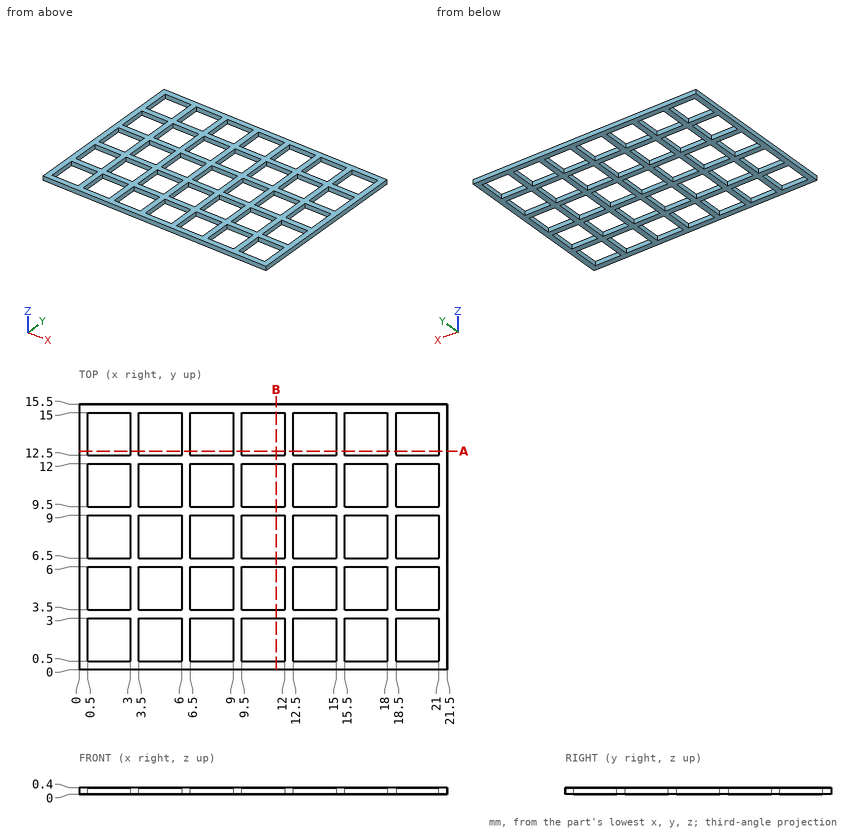
Input: dimensioned drawing with shaded views. Units: mm. Origin: part minimum x, y, z. Round coordinates to 2 decimals unless told otherwise and drop trailing zeros. Order: outer loops, then holes, each group sorted by start corner. A loop starts at its lowest first (then second) coordinate and runs counter-clockwise, first axis right, second up. Notation, with made-up numbers: (37.25, 0) -> (44.25, 0) arc R19 cw to (44.25, 5) -> close; hole circle Ø9 at (-3.5, 22). An arc over 180 degrees is marked (long way). Put each result on its own line as item: value. Start each with the question number.
Q1. Line query: probe 1 along Y at (x, z) = (5, 0.25). Output: solid intervals per line, ascending.
Q2. Section A-A on y = 12.75. Give the number of separate pieces and of enclosed holes in the cut face, and give its area (3 significant figures).
Q3. Section B-B on x = 11.5. Return the cut outline in (y, z), and give its area (3 significant figures).
Ans:
1. probe 1: y = 0 to 0.5, 3 to 3.5, 6 to 6.5, 9 to 9.5, 12 to 12.5, 15 to 15.5
2. separate pieces: 8
2. enclosed holes: 0
2. area: 1.60 mm2
3. outline: (0, 0) -> (0.5, 0) -> (0.5, 0.4) -> (0, 0.4) -> close; (3, 0) -> (3.5, 0) -> (3.5, 0.4) -> (3, 0.4) -> close; (6, 0) -> (6.5, 0) -> (6.5, 0.4) -> (6, 0.4) -> close; (9, 0) -> (9.5, 0) -> (9.5, 0.4) -> (9, 0.4) -> close; (12, 0) -> (12.5, 0) -> (12.5, 0.4) -> (12, 0.4) -> close; (15, 0) -> (15.5, 0) -> (15.5, 0.4) -> (15, 0.4) -> close
3. area: 1.20 mm2
